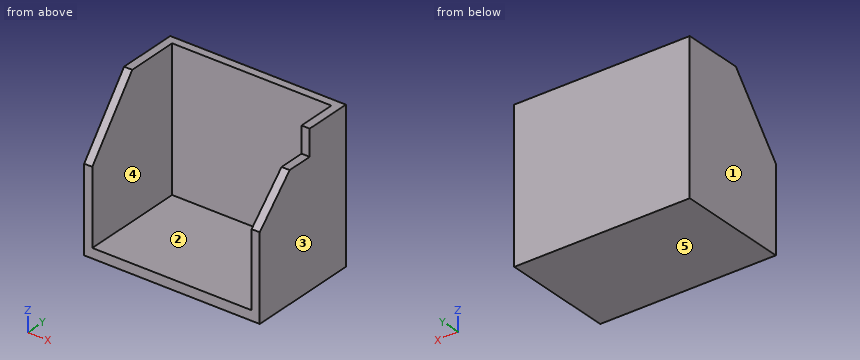
Autodesk Fusion 360 part; units mm, degrees
sketch "Sketch1" plane through (0, 0, 0) normal (0, 0, 1) x (1, 0, 0)
  line L0 (0, 0) -> (49, 0)
  line L1 (49, 0) -> (49, 32)
  line L2 (49, 32) -> (0, 32)
  line L3 (0, 32) -> (0, 0)
  line L4 (0, 0) -> (-2.5, 0)
  line L5 (-2.5, 0) -> (51.5, 0)
  line L6 (51.5, 0) -> (51.5, 34.5)
  line L7 (51.5, 34.5) -> (-2.5, 34.5)
  line L8 (-2.5, 34.5) -> (-2.5, 0)
  dimension "d1" = 49
  dimension "d2" = 32
  dimension "d3" = 2.5
  dimension "d4" = 34.5
  dimension "d5" = 54
extrude "Extrude1" add sketch "Sketch1" against normal blind 3
sketch "Sketch2" plane through (0, 0, 0) normal (0, 1, 0) x (1, 0, 0)
extrude "Extrude2" add sketch "Sketch1" along normal blind 43 contours L1 L2 L3 L4 L5 L6 L7 L8
sketch "Sketch3" plane through (51.5, 0, 0) normal (1, 0, 0) x (0, 1, 0)
  line L0 (0, 43) -> (0, -3)
  line L1 (0, -3) -> (34.5, -3)
  line L2 (34.5, -3) -> (34.5, 43)
  line L3 (34.5, 43) -> (0, 43)
  line L4 (34.5, 43) -> (32, 43)
  line L5 (32, 43) -> (0, 43)
  line L6 (0, 43) -> (16, 43)
  line L7 (16, 43) -> (12, 43)
  line L8 (12, 43) -> (12, 35)
  line L9 (12, 35) -> (16, 35)
  line L10 (16, 35) -> (16, 43)
  line L11 (16, 43) -> (20, 43)
  line L12 (20, 43) -> (20, 35)
  line L13 (20, 35) -> (16, 35)
  line L14 (16, 35) -> (16, 43)
  point P0 (32, 43)
  point P1 (32, 43)
  dimension "d10" = 4
  dimension "d11" = 8
  dimension "d12" = 8
extrude "Extrude3" cut sketch "Sketch3" against normal blind 10 contours L3 L5 L6 L7 L8 L9 L10 L14 | L3 L5 L10 L11 L12 L13 L14
sketch "Sketch4" plane through (51.5, 0, 0) normal (1, 0, 0) x (0, 1, 0)
  line L0 (20, 43) -> (20, 35)
  line L1 (20, 35) -> (12, 35)
  line L2 (12, 35) -> (12, 43)
  line L3 (12, 43) -> (0, 43)
  line L4 (0, 43) -> (0, -3)
  line L5 (0, -3) -> (34.5, -3)
  line L6 (34.5, -3) -> (34.5, 43)
  line L7 (34.5, 43) -> (20, 43)
  line L8 (0, 43) -> (0, 23)
  line L9 (0, 23) -> (12, 35)
  dimension "d15" = 20
extrude "Extrude4" cut sketch "Sketch4" against normal blind 5 contours L2 L3 L4 L8 L9
sketch "Sketch5" plane through (-2.5, 0, 0) normal (-1, 0, 0) x (0, -1, 0)
  line L0 (-34.5, 43) -> (-34.5, -3)
  line L1 (-34.5, -3) -> (0, -3)
  line L2 (0, -3) -> (0, 43)
  line L3 (0, 43) -> (-34.5, 43)
  line L4 (0, 43) -> (-16, 43)
  line L5 (0, 43) -> (0, 23)
  line L6 (-16, 43) -> (0, 23)
  dimension "d18" = 16
  dimension "d19" = 20
extrude "Extrude5" cut sketch "Sketch5" against normal blind 10 contours L2 L3 L4 L5 L6
Design review of the part built by this model. Coordinates are the model's own, in mm. Face numbers are marked on the shaded views. A direction names the side the tool comes from. Give positions to 0.01 mm unless a question says otherwise; leave off trailing zeros. Loops run counter-clockwise (first coordinate to the right, second up) from the corner with the lowest first, then second, coordinate; pieces in that order, holes last. Notation, with made-up numbers: (-35, 14.5) -> (9, 14.5) arc R23 ccw to (9, 34.5) -> close; hole circle Ø4 at (-38.75, 58). An arc over 180 degrees is marked (long way). One line per item, written item: value.
Q1. For L1, parallel to X at y = 25, z = 10; L2, parallel to Y at x = 19, z = 28; L3, parallel to Z at x = 20, y = 7, list the stretches that pass through material, from the lowest coordinate up.
Numbers:
L1: x = -2.5 to 0, 49 to 51.5
L2: y = 32 to 34.5
L3: z = -3 to 0
Q2. Draft analysis for pull direction X (two halves, no side actions). For the marked faces 1, 2 and 3, state which applies: pulls with the +X half, pulls with the -X half, needs draft (parallel to the pull), parting line crosses it, or undercut.
Numbers:
face 1: pulls with the -X half
face 2: undercut
face 3: pulls with the +X half
Q3. For pin 1 Ø8 at (x, y) = (17, 10) entering from +Z; pin 2 Ø0.8 at (x, y) = (50.5, 17) entering from +Z; pin 3 Ø0.8 at (x, z) = (50, 40) entering from -Y, all flat-tipped, find the tip position at first contact; note any pin that passes through.
Numbers:
pin 1: stops at z = 0
pin 2: stops at z = 35
pin 3: stops at y = 20
Q4. We need section C-C on y = 2. Give the boundary of the cut face in (x, z), and give its area (3 significant figures).
Numbers:
outline: (-2.5, -3) -> (51.5, -3) -> (51.5, 25) -> (49, 25) -> (49, 0) -> (0, 0) -> (0, 25.5) -> (-2.5, 25.5) -> close
area: 288 mm^2
Q5. We need section A-A on z = 17.5. Give the boundary of the cut face in (x, y).
Numbers:
outline: (-2.5, 0) -> (0, 0) -> (0, 32) -> (49, 32) -> (49, 0) -> (51.5, 0) -> (51.5, 34.5) -> (-2.5, 34.5) -> close
Q6. We need section B-B on x = 41.5. Give the boundary of the cut face in (y, z).
Numbers:
outline: (0, -3) -> (34.5, -3) -> (34.5, 43) -> (32, 43) -> (32, 0) -> (0, 0) -> close
Q7. Machinability: for the marked faces 4 and 5, which of the approach directions +Z, -Z, +X, -X, +Y, -Y give a long, thin tool a straight path to every point of the face, cutting with its end or side? Answer none if there is none.
Numbers:
face 4: +Z, -Y
face 5: -Z, +X, -X, +Y, -Y
